Work out the finished part from the listing and answer in its coordinate system (mm). Face numbers are marked on the shaded views. A direction names the side the tool comes from. Give positions to 0.01 mm unless a question says otherwise; leave off trailing zeros. Write each loop counter-clockwise with the first axis right and the second up, starting at its lowest first coordinate (ties: lowest second). Pieces come first, ordered by that corner, then holes. Notation, with made-up numbers: (64.5, 12) -> (111.5, 12) arc R14 cw to (111.5, 39) -> close; hole circle Ø3 at (68.25, 32). An arc over 180 degrees is marked (long way). Use a Markdown table: item, result. Add a question column.
Q1. Each of these flat-tipped pins is pushed along its axis until it touches: pin 1 Ø12 at (y, z) = (81, -199.5) entering from +X; pin 2 Ø6 at (x, z) = (-140, -206) entering from -Y; pin 3 Ø12 at (y, z) = (122.5, -186.5) entering from -X; pin 4 Ø10 at (x, z) = (-129, -202) entering from -Y. Where does it stop, or does it pass through?
Q2. Section B-B, the plane x = -104 is taken. Give the vertices of the cut face in (y, z) (3 decimals), plus the area to 3 significant figures.
Q3. Section A-A, the plane x = -123.5 is taken. Give the vertices of the cut face in (y, z), plus the area to 3 significant figures.
Q4. For the marked faces 4 and 5, determine the directions among +Z, -Z, +X, -X, +Y, -Y from which every point of the face is accessible in a straight line to the end or side of a thin tool.
Q5. For a pull along X with two mould halves and no side action, classify the marked faces 1, 2 and 3 as pulls with the +X half, pulls with the -X half, needs draft (parallel to the pull), parting line crosses it, or undercut.
Q6. Consider line 1 (X direction, y = 37, z = -195.5); line 2 (X direction, y = 40.5, z = -206); line 3 (X direction, y = 129.5, z = -217.5). Determine where each line is inside the solid, lowest interval first.
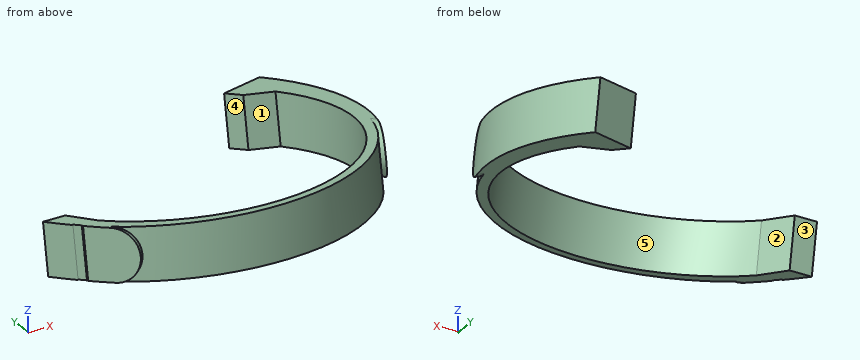
Autodesk Inventor part; units mm, degrees
ref_plane "YZ Plane" through (0, 0, 0) normal (1, 0, 0) x (0, 1, 0)
ref_plane "XZ Plane" through (0, 0, 0) normal (0, 1, 0) x (-1, 0, 0)
ref_plane "Work Plane1" through (27.2016, 137.7902, -207.6153) normal (0, 0, 1) x (1, 0, 0)
ref_plane "Work Plane2" through (-81.5141, 115.844, -101.5145) normal (0, 0, 1) x (1, 0, 0)
sketch "Sketch2" plane through (27.2016, 137.7902, -207.6153) normal (0, 0, 1) x (1, 0, 0)
  line L0 (-50.9279, -141.1381) -> (10.2073, -141.1381)
  point P0 (-27.2016, -137.7902)
ref_plane "Work Plane4" through (-23.7263, -2.2452, -201.3618) normal (0, 0.1736482, 0.9848078) x (1, 0, 0)
ref_plane "Work Plane3" through (-23.7263, -3.3479, -207.6153) normal (0, 0.1736482, 0.9848078) x (1, 0, 0)
sketch "Sketch1" plane through (-81.5141, 95.2083, -218.5455) normal (0, 0.1736482, 0.9848078) x (1, 0, 0)
  line L0 (120.3524, 26.6103) -> (110.8538, 39.0511)
  line L1 (109.9403, 39.2699) -> (118.8077, 27.6558)
  line L2 (117.4827, 25.3957) -> (118.8077, 27.6558)
  line L3 (108.6153, 37.0098) -> (109.9403, 39.2699)
  line L4 (-70.1644, -17.8234) -> (-70.1644, -42.3865)
  line L5 (-67.5144, -23.0328) -> (-67.5144, -49.6797)
  line L6 (-7.2549, -88.8185) -> (-7.2549, -90.7022)
  line L7 (88.6474, -22.0445) -> (90.1001, -24.6815)
  arc A0 (90.1001, -24.6815) -> (85.4909, 74.1551) centre (-2.6058, 20.521) ccw
  line L8 (68.6883, 59.486) -> (92.8567, 47.8109)
  ellipse E0 centre (117.3159, 24.5297) end of major axis (77.6327, 47.7943) minor radius 6.9177 (109.5288, 36.791) -> (89.1504, 46.193) ccw
  ellipse E1 centre (118.6409, 26.7898) end of major axis (80.226, 49.3108) minor radius 6.6966 (109.9403, 39.2699) -> (91.8991, 47.566) ccw
  line L9 (120.3524, 26.6103) -> (110.8538, 39.0511)
  line L10 (120.3524, 26.6103) -> (110.8538, 39.0511)
  line L11 (-70.1644, -47.9895) -> (-70.1644, -41.1809)
  line L12 (-78.1686, -54.9211) -> (-78.1686, -34.8)
  line L13 (-78.1686, -34.8) -> (-78.1686, -33.261)
  ellipse E2 centre (-68.1686, -34.8) end of major axis (-78.1686, -34.8) minor radius 8.1116 (-75.6686, -29.4347) -> (-78.1686, -34.8) ccw
  line L14 (-78.1686, -54.9211) -> (-78.1686, -34.8)
  line L15 (-77.6379, -18.1276) -> (-66.4488, -18.1276)
  line L16 (-66.4488, -18.1276) -> (-58.9889, -34.0305)
  arc A1 (-77.6379, -18.1276) -> (-51.8229, -55.9602) centre (98.8915, 74.6035) ccw
  line L17 (-51.8229, -55.9602) -> (-49.6664, -53.6662)
  ellipse E3 centre (43.7773, 28.2672) end of major axis (9.3333, 77.3077) minor radius 54.627 (86.8491, 61.886) -> (73.2137, 75.1203) ccw
  ellipse E4 centre (87.3016, 57.9812) end of major axis (48.0133, 78.9413) minor radius 0.2829 (58.2062, 73.2871) -> (75.8706, 63.7724) ccw
  ellipse E5 centre (86.0543, 55.6432) end of major axis (46.766, 76.6033) minor radius 0.2829 (56.9589, 70.9491) -> (74.6233, 61.4344) ccw
  ellipse E6 centre (-82.1686, -42.8548) end of major axis (-78.1686, -42.8548) minor radius 0.6946 (-78.1686, -42.8548) -> (-82.1686, -42.1602) ccw
  line L18 (85.4909, 74.1551) -> (63.6157, 67.3502)
  arc A2 (-66.1246, -22.0445) -> (76.0856, 61.886) centre (8.3655, 14.1852) ccw
  arc A3 (-70.1644, -30.1049) -> (79.8851, 69.6106) centre (7.0855, 16.4044) ccw
  line L19 (63.6157, 67.3502) -> (68.6883, 59.486)
  point P0 (81.5141, -131.7119)
  point P1 (-70.1644, -31.1405)
  point P2 (97.5203, 45.2683)
  point P3 (-67.5144, -35.2635)
  point P4 (96.3482, 45.7746)
  point P5 (98.1827, 42.4146)
  point P6 (110.3672, 38.7108)
  point P7 (-70.1644, -18.1276)
  point P8 (81.3429, 53.3729)
  point P9 (-67.5144, -34.2466)
extrude "Extrusion1" add sketch "Sketch1" along normal blind 25.4 contours E0 A3 E3 L18 A0 | A0 L7 A3 E0 | A3 L4 L15 L16 A2 L8 | L8 L19 L18 E3 A3 | L17 A1 L5 A3 | L4 A1 L15
fillet "Fillet1" radius 12.7 4 edges at (7.8596, 76.6109, -189.4744) (7.8596, 72.2002, -214.4886) (-132.2588, 41.2279, -209.0273) (-132.2588, 45.6386, -184.0132)
properties part number "thigh_strap_03"
Result set:
| question | item | result |
|---|---|---|
| 1 | pin 1 | stops at x = 13.99 |
| 1 | pin 2 | stops at y = 44.98 |
| 1 | pin 3 | passes through |
| 1 | pin 4 | stops at y = 38.19 |
| 2 | outline | (27.474, -206.602) -> (33.472, -207.66) -> (37.883, -182.646) -> (31.885, -181.588) -> close |
| 2 | area | 155 mm2 |
| 3 | outline | (36.86, -208.26) -> (44.4, -209.59) -> (48.81, -184.57) -> (41.28, -183.24) -> close |
| 3 | area | 194 mm2 |
| 4 | face 4 | +Z, -X |
| 4 | face 5 | none |
| 5 | face 1 | pulls with the -X half |
| 5 | face 2 | undercut |
| 5 | face 3 | needs draft |
| 6 | line 1 | x = -120.13 to -107.2, -39.1 to -28.73 |
| 6 | line 2 | x = -128.1 to -117.05, -29.24 to -20.76 |
| 6 | line 3 | x = 7.38 to 18.19 |
